The listing builds one solid part. Answer for the finished solid, in the listing's coordinates (mm). A direction names the side the tool comes from. Round coordinates to 2 decimals unless told otherwise and drop trailing zeros. Loops run counter-clockwise (first coordinate to the right, second up) from the corner with the lowest first, then second, coordinate; pieces in that order, holes last. Notation, with made-up numbers: (-14.5, -16) - (40.5, -16) arc R20 cw to (40.5, 2) - close; hole circle Ø7 at (35, 30). An arc over 180 degrees is marked (long way). Write item = value, one per line. Start each with the question number.
1) Section D-D, the plane z = 2 is taken. Determine the outline of the cut face in (x, y) (3 decimals), and give its area (3 significant figures).
2) Section A-A, the plane x = -10.25 is taken. Determine the outline of the cut face in (y, z) (3 decimals).
3) Section B-B, the plane x = -0.75 is taken. Determine the outline of the cut face in (y, z) (3 decimals), and give its area (3 significant figures).
4) Section C-C, the plane y = -2.75 is taken. Determine the outline of the cut face in (x, z) (3 decimals).
5) For a pull along Y with two mould halves and no side action, classify faces 1 (the flat face through (-6, -3.175, 0)), 2 (the flat face through (-12.7, 0, 1.4)), 3 (the flat face through (-2, -1, 0.794)) as released by +Y, released by -Y, zero draft, split by the parting line, or undercut.
6) Straight lines are drawn through the part: line 1 along Y through (x, z) = (-8.5, 0) (3 decimals); line 2 along Z through (x, y) = (2.25, -0.75). For each, find the intervals that lie inside material, in ascending order.
7) Given pin 1 Ø1.9 at (x, y) = (1, 0) entering from -Z; pin 2 Ø1 at (x, z) = (0, 2) entering from -Y; pin 3 Ø3 at (x, y) = (1, -1) entering from +Z, each flat-ended and moving along its own axis, determine where each tip first touches the part or whether it passes through.
8) A tool of negligible diameter and unlimited length cuts with its end or side. For faces 4 (the cylindrical face through (-3.43, 0.06, 2)), 5 (the cylindrical face through (-3.43, 0.06, -1.97)), 6 (the cylindrical face through (-8.386, -1.103, 0.245)), from which of +Z, -Z, +X, -X, +Y, -Y can it reach the whole face along a straight path? Write none if from no direction.
from build123d import *

# Parameters (mm, degrees)
BOSS_EXTRUDE2_DEPTH              = 0.79375
SKETCH4_W                        = 6.35
SKETCH4_H                        = 6.35
BOSS_EXTRUDE3_DEPTH              = 6.35
BOSS_EXTRUDE4_DEPTH              = 3.175
F_4_40_TAPPED_HOLE3_D            = 2.2606
F_4_40_TAPPED_HOLE3_DEPTH        = 8.509
F_4_40_TAPPED_HOLE3_TIP          = 0.679152758
F_1_8_0_125_DIAMETER_HOLE1_D     = 3.175
F_1_8_0_125_DIAMETER_HOLE1_DEPTH = 1.5875


with BuildPart() as part:
    # Sketch2 → Boss-Extrude2 (new body, symmetric)
    with BuildSketch(Plane.XY):
        with BuildLine():
            Line((-6.35, 3.175), (0, 3.175))
            ThreePointArc((0, 3.175), (3.175, 0), (0, -3.175))
            Line((0, -3.175), (-6.35, -3.175))
            Line((-6.35, -3.175), (-6.35, 3.175))
        make_face()
    extrude(amount=BOSS_EXTRUDE2_DEPTH, both=True)

    # Sketch4 → Boss-Extrude3 (add)
    with BuildSketch(Plane.ZY.offset(6.35)):
        Rectangle(SKETCH4_W, SKETCH4_H)
    extrude(amount=BOSS_EXTRUDE3_DEPTH)

    # Sketch10 → Boss-Extrude4 (add, symmetric)
    with BuildSketch(Plane.XY):
        with BuildLine():
            Line((-6.35, 3.175), (-3.175, 3.175))
            Line((-3.175, 3.175), (-1.295150956, 3.175))
            ThreePointArc((-1.295150956, 3.175), (-3.429, 0), (-1.295150956, -3.175))
            Line((-1.295150956, -3.175), (-3.175, -3.175))
            Line((-3.175, -3.175), (-6.35, -3.175))
            Line((-6.35, -3.175), (-6.35, 3.175))
        make_face()
    extrude(amount=BOSS_EXTRUDE4_DEPTH, both=True)

    # #4-40 Tapped Hole3
    with Locations(Plane.ZY.offset(12.7)):
        with Locations((0, 0)):
            Hole(F_4_40_TAPPED_HOLE3_D / 2, depth=F_4_40_TAPPED_HOLE3_DEPTH)
            with Locations((0, 0, -(F_4_40_TAPPED_HOLE3_DEPTH + F_4_40_TAPPED_HOLE3_TIP / 2))):  # 118° drill point
                Cone(0, F_4_40_TAPPED_HOLE3_D / 2, F_4_40_TAPPED_HOLE3_TIP, mode=Mode.SUBTRACT)

    # 1/8 (0.125) Diameter Hole1
    with Locations(Plane.XY.offset(0.79375)):
        with Locations((0, 0)):
            Hole(F_1_8_0_125_DIAMETER_HOLE1_D / 2, depth=F_1_8_0_125_DIAMETER_HOLE1_DEPTH)


solid = part.part
Geometry check:
q1.outline = (-12.7, -3.175) - (-1.295, -3.175) arc R3.429 cw to (-1.295, 3.175) - (-12.7, 3.175) - close
q1.area = 62.6 mm2
q2.outline = (-3.175, -3.175) - (3.175, -3.175) - (3.175, 3.175) - (-3.175, 3.175) - close; hole circle Ø2.261 at (0, 0)
q3.outline = (-3.175, -0.794) - (-1.399, -0.794) - (-1.399, 0.794) - (-3.175, 0.794) - close; (1.399, -0.794) - (3.175, -0.794) - (3.175, 0.794) - (1.399, 0.794) - close
q3.area = 5.64 mm2
q4.outline = (-12.7, -3.175) - (-2.048, -3.175) - (-2.048, -0.794) - (1.587, -0.794) - (1.587, 0.794) - (-2.048, 0.794) - (-2.048, 3.175) - (-12.7, 3.175) - close
q5.face_1 = released by -Y
q5.face_2 = zero draft
q5.face_3 = undercut
q6.line_1 = -3.175 to -1.13, 1.13 to 3.175
q6.line_2 = -0.79 to 0.79
q7.pin_1 = -0.79
q7.pin_2 = through
q7.pin_3 = 0.79
q8.face_4 = +Z, +X
q8.face_5 = -Z, +X
q8.face_6 = -X
